For this review, take the finished solid that the model builds, in its own axes (mm). A direction names the side the tool comes from. Coordinates: 2 decimals unless noted, no trailing zeros. Order: outer loops, then holes, each group sorted by start corner. A loop starts at its lowest first (then second) coordinate and runs counter-clockwise, first axis right, second up.
from build123d import *

# Parameters (mm, degrees)
SKETCH1_R           = 14
BOSS_EXTRUDE1_DEPTH = 19.1
SKETCH1_3_R         = 4.5
SKETCH1_3_R_2       = 2.5
BOSS_EXTRUDE2_DEPTH = 1.7
BOSS_EXTRUDE4_DEPTH = 2.3
BOSS_EXTRUDE5_DEPTH = 9.5
BOSS_EXTRUDE6_DEPTH = 2.3
SKETCH1_9_R         = 1.75
BOSS_EXTRUDE7_DEPTH = 1


with BuildPart() as part:
    # Sketch1 → Boss-Extrude1 (new body)
    with BuildSketch(Plane.XY):
        Circle(SKETCH1_R)
    extrude(amount=BOSS_EXTRUDE1_DEPTH)

    # Sketch1_3 → Boss-Extrude2 (add)
    with BuildSketch(Plane.XY):
        with Locations((0.027687475, 7.999952088)):
            Circle(SKETCH1_3_R)
        with Locations((0.027687475, 7.999952088)):
            Circle(SKETCH1_3_R_2, mode=Mode.SUBTRACT)
    extrude(amount=-BOSS_EXTRUDE2_DEPTH)

    # Sketch1_6 → Boss-Extrude4 (add)
    with BuildSketch(Plane.XY):
        with BuildLine():
            Line((-1.972312525, 9.499952088), (0.027687475, 9.499952088))
            Line((0.027687475, 9.499952088), (2.027687475, 9.499952088))
            ThreePointArc((2.027687475, 9.499952088), (0.027687475, 10.499952088), (-1.972312525, 9.499952088))
        make_face()
    extrude(amount=-BOSS_EXTRUDE4_DEPTH)

    # Sketch1_7 → Boss-Extrude5 (add)
    with BuildSketch(Plane.XY):
        with BuildLine():
            Line((2.027687475, 9.499952088), (0.027687475, 9.499952088))
            Line((0.027687475, 9.499952088), (0.027687475, 6.499952088))
            Line((0.027687475, 6.499952088), (2.027687475, 6.499952088))
            ThreePointArc((2.027687475, 6.499952088), (2.39939572, 7.209382673), (2.527687475, 7.999952088))
            ThreePointArc((2.527687475, 7.999952088), (2.39939572, 8.790521503), (2.027687475, 9.499952088))
        make_face()
        with BuildLine():
            Line((0.027687475, 6.499952088), (0.027687475, 9.499952088))
            Line((0.027687475, 9.499952088), (-1.972312525, 9.499952088))
            ThreePointArc((-1.972312525, 9.499952088), (-2.472312525, 7.999952088), (-1.972312525, 6.499952088))
            Line((-1.972312525, 6.499952088), (0.027687475, 6.499952088))
        make_face()
    extrude(amount=-BOSS_EXTRUDE5_DEPTH)

    # Sketch1_8 → Boss-Extrude6 (add)
    with BuildSketch(Plane.XY):
        with BuildLine():
            Line((2.027687475, 6.499952088), (0.027687475, 6.499952088))
            Line((0.027687475, 6.499952088), (-1.972312525, 6.499952088))
            ThreePointArc((-1.972312525, 6.499952088), (0.027687475, 5.499952088), (2.027687475, 6.499952088))
        make_face()
    extrude(amount=-BOSS_EXTRUDE6_DEPTH)

    # Sketch1_9 → Boss-Extrude7 (add)
    # profile 1 of 2: a face of its own
    with BuildSketch(Plane.XY):
        with BuildLine():
            Line((-13.564798107, 3.46356064), (-18.003733752, 3.46356064))
            ThreePointArc((-18.003733752, 3.46356064), (-21, 0), (-18.003733752, -3.46356064))
            Line((-18.003733752, -3.46356064), (-13.564798107, -3.46356064))
            ThreePointArc((-13.564798107, -3.46356064), (-14, 0), (-13.564798107, 3.46356064))
        make_face()
        with Locations((-17.5, 0)):
            Circle(SKETCH1_9_R, mode=Mode.SUBTRACT)
    # profile 2 of 2: a face of its own
    with BuildSketch(Plane.XY):
        with BuildLine():
            Line((17.527687475, 3.46356064), (13.564798107, 3.46356064))
            ThreePointArc((13.564798107, 3.46356064), (13.89077344, 1.745397734), (14, 0))
            ThreePointArc((14, 0), (13.89077344, -1.745397734), (13.564798107, -3.46356064))
            Line((13.564798107, -3.46356064), (17.527687475, -3.46356064))
            ThreePointArc((17.527687475, -3.46356064), (20.991248115, 0), (17.527687475, 3.46356064))
        make_face()
        with Locations((17.527687475, 0)):
            Circle(SKETCH1_9_R, mode=Mode.SUBTRACT)
    extrude(amount=BOSS_EXTRUDE7_DEPTH)


solid = part.part
1. Take a section at B-B, the plane y = 0. Give the boundary of the cut face in (x, z).
Answer below:
outline: (-21, 0) - (-19.25, 0) - (-19.25, 1) - (-21, 1) - close; (-15.75, 0) - (15.78, 0) - (15.78, 1) - (14, 1) - (14, 19.1) - (-14, 19.1) - (-14, 1) - (-15.75, 1) - close; (19.28, 0) - (20.99, 0) - (20.99, 1) - (19.28, 1) - close
2. The part is to be moulded in two halves that separate along X. For faces 1 (the face through (0, 0, 0)), 2 (the face through (13.35, 4.21, 9.42)), 3 (the face through (16.139, -1.065, 0.493)), say which applies: +X half, -X half, draft (parallel to the pull), parting line (faces both ways), or undercut.
Answer below:
face 1: draft
face 2: parting line
face 3: undercut
3. Take a section at C-C, the plane x = 0. Give the boundary of the cut face in (y, z).
Answer below:
outline: (-14, 0) - (3.5, 0) - (3.5, -1.7) - (5.5, -1.7) - (5.5, -2.3) - (6.5, -2.3) - (6.5, -9.5) - (9.5, -9.5) - (9.5, -2.3) - (10.5, -2.3) - (10.5, -1.7) - (12.5, -1.7) - (12.5, 0) - (14, 0) - (14, 19.1) - (-14, 19.1) - close
4. To check wall thickness, follow L1, parallel to Y at x = -17.5, z = 0.2; L2, parallel to Z at x = -7, y = -7.5; L3, parallel to Y at x = -0.5, z = 10. State the ranges of each line that lie inside material, in increasing order.
Answer below:
L1: y = -3.46 to -1.75, 1.75 to 3.46
L2: z = 0 to 19.1
L3: y = -13.99 to 13.99
5. Take a section at A-A, the plane x = -17.5. Give the boundary of the cut face in (y, z).
Answer below:
outline: (-3.46, 0) - (-1.75, 0) - (-1.75, 1) - (-3.46, 1) - close; (1.75, 0) - (3.46, 0) - (3.46, 1) - (1.75, 1) - close
6. Take a section at D-D, the plane z = -5.25. Give the boundary of the cut face in (x, y), plus the area to 3 significant figures.
Answer below:
outline: (-1.97, 6.5) - (2.03, 6.5) arc R2.5 ccw to (2.03, 9.5) - (-1.97, 9.5) arc R2.5 ccw to start
area: 14.0 mm2
7. Machinability: for faces 4 (the face through (15.6, 3.464, 0.5)), 5 (the face through (0, 9.5, -6)), 6 (the face through (15.5, -3.464, 0.5)), 7 (the face through (0, 6.5, -6)), which of the approach directions +Z, -Z, +X, -X, +Y, -Y give a long, thin tool a straight path to every point of the face, cutting with its end or side? Answer none if there is none.
Answer below:
face 4: +Z, -Z, +X, +Y
face 5: -Z, +X, -X, +Y
face 6: +Z, -Z, +X, -Y
face 7: -Z, +X, -X, -Y
8. Clearance check with flat-ended pins moving along their axes: pin 1 Ø4 at (y, z) = (-5, 10.5) entering from -X; pin 2 Ø4 at (x, y) = (17.53, 0) entering from -Z; pin 3 Ø3 at (x, z) = (-0.5, -7) entering from -Y. State where each tip first meets the part, or that it passes through.
Answer below:
pin 1: stops at x = -13.67
pin 2: stops at z = 0
pin 3: stops at y = 6.5
